```python
from build123d import *

# Parameters (mm, degrees)
SKETCH_1_R          = 11.5
SKETCH_1_R_2        = 1.5
EXTRUDE_1_DEPTH     = 3
SKETCH_2_R          = 5.25
EXTRUDE_2_DEPTH     = 3
CUT_EXTRUDE_1_DEPTH = 4.5
CUT_EXTRUDE_2_REACH = 3.5
SKETCH_4_R          = 1.65


with BuildPart() as part:
    # 草圖1 → 填料-伸長1 (new body)
    with BuildSketch(Plane.XY):
        Circle(SKETCH_1_R)
        with Locations((0, 8)):
            Circle(SKETCH_1_R_2, mode=Mode.SUBTRACT)
        with Locations((8, 0)):
            Circle(SKETCH_1_R_2, mode=Mode.SUBTRACT)
        with Locations((0, -8)):
            Circle(SKETCH_1_R_2, mode=Mode.SUBTRACT)
        with Locations((-8, 0)):
            Circle(SKETCH_1_R_2, mode=Mode.SUBTRACT)
    extrude(amount=EXTRUDE_1_DEPTH)

    # 草圖2 → 填料-伸長2 (add)
    with BuildSketch(Plane.XY.offset(3)):
        Circle(SKETCH_2_R)
    extrude(amount=EXTRUDE_2_DEPTH)

    # 草圖3 → 除料-伸長1 (cut)
    with BuildSketch(Plane.XY.offset(6)):
        Polygon((2.886751346, 0), (1.443375673, 2.5), (-1.443375673, 2.5), (-2.886751346, 0), (-1.443375673, -2.5), (1.443375673, -2.5), align=None)
    extrude(amount=-CUT_EXTRUDE_1_DEPTH, mode=Mode.SUBTRACT)

    # 草圖4 → 除料-伸長2 (cut, up to next)
    with BuildSketch(Plane.XY.offset(1.5), mode=Mode.PRIVATE) as cut_extrude_2_sk1:
        Circle(SKETCH_4_R)
    cut_extrude_2_tool1 = extrude(cut_extrude_2_sk1.sketch, amount=-CUT_EXTRUDE_2_REACH, mode=Mode.PRIVATE) & part.part
    add(cut_extrude_2_tool1.solids().sort_by_distance((0, 0, 1.5))[0], mode=Mode.SUBTRACT)


solid = part.part
```
Here's how the part is built. I have some questions about the finished solid (model axes, mm). A direction names the side the tool comes from. Coordinates: 2 decimals unless noted, no trailing zeros. Loops run counter-clockwise (first coordinate to the right, second up) from the corner with the lowest first, then second, coordinate; pieces in that order, holes last. Notation, with made-up numbers: (-28.5, 36.5) - (24.5, 36.5) arc R29 ccw to (24.5, 67.5) - close; hole circle Ø2 at (18.25, -6). An arc over 180 degrees is marked (long way). Answer as CSV lines item,"result".
Q1. If we section it at C-C, the plane x = -8.75: Write out the boundary of the cut face in (y, z), and give its area (3 significant figures).
Response:
outline,"(-7.46, 0) - (-1.3, 0) - (-1.3, 3) - (-7.46, 3) - close; (1.3, 0) - (7.46, 0) - (7.46, 3) - (1.3, 3) - close"
area,"37.0 mm2"
Q2. For pin 1 (0.9 mm diameter, centred on x = 0, z = 3.5, fed in from +Y); pin 2 (0.9 mm diameter, centred on x = 0, z = 4, fed in from -Y); pin 3 (2 mm diameter, centred on x = -4, z = 1.5, fed in from +Y); pin 4 (2.5 mm diameter, centred on x = 0, y = 8, fed in from -Z), each with a flat end and sliding along its axis, tell me the tip position at first contact or that it passes through.
Response:
pin 1,"y = 5.25"
pin 2,"y = -5.25"
pin 3,"y = 11.1"
pin 4,"through"
Q3. If we section it at A-A, the plane x = 0: Write out the boundary of the cut face in (y, z).
Response:
outline,"(-11.5, 0) - (-9.5, 0) - (-9.5, 3) - (-11.5, 3) - close; (-6.5, 0) - (-1.65, 0) - (-1.65, 1.5) - (-2.5, 1.5) - (-2.5, 6) - (-5.25, 6) - (-5.25, 3) - (-6.5, 3) - close; (1.65, 0) - (6.5, 0) - (6.5, 3) - (5.25, 3) - (5.25, 6) - (2.5, 6) - (2.5, 1.5) - (1.65, 1.5) - close; (9.5, 0) - (11.5, 0) - (11.5, 3) - (9.5, 3) - close"
Q4. We'd pull the mould along X, two halves only. Please class faces 1 (the face through (-1.5, 11.4, 1.5)), 2 (the face through (-9.5, 0.07, 1.48)), 3 (the face through (-2.4, 1.2, 6)): pulls with the +X half, pulls with the -X half, needs draft (parallel to the pull), parting line crosses it, or undercut.
Response:
face 1,"parting line crosses it"
face 2,"undercut"
face 3,"needs draft"
Q5. If we section it at B-B, the plane y = -8: Write out the boundary of the cut face in (x, z).
Response:
outline,"(-8.26, 0) - (-1.5, 0) - (-1.5, 3) - (-8.26, 3) - close; (1.5, 0) - (8.26, 0) - (8.26, 3) - (1.5, 3) - close"
Q6. If we section it at D-D, the plane z = 4.65: Write out the boundary of the cut face in (x, y).
Response:
outline,"circle Ø10.5 at (0, 0); hole (-2.89, 0) - (-1.44, -2.5) - (1.44, -2.5) - (2.89, 0) - (1.44, 2.5) - (-1.44, 2.5) - close"
Q7. For faces 4 (the face through (-1.216, 1.115, 0.76)), 5 (the face through (5, 1.6, 4.5)), which set-ups out of +Z, -Z, +X, -X, +Y, -Y let a thin tool reach every point of the face, with its end or its side?
Response:
face 4,"+Z, -Z"
face 5,"+Z"
Q8. If I drill on L1, parallel to Y at x = 0, z = 1.05; L2, parallel to X at y = 0.75, z = 1.65; L3, parallel to Z at x = 0.5, y = 9.5, over which ranges is the centre line in solid material (lowest first)? Write a range as [from, to].
Response:
L1,"[-11.5, -9.5], [-6.5, -1.65], [1.65, 6.5], [9.5, 11.5]"
L2,"[-11.48, -9.3], [-6.7, -2.45], [2.45, 6.7], [9.3, 11.48]"
L3,"[0, 3]"
